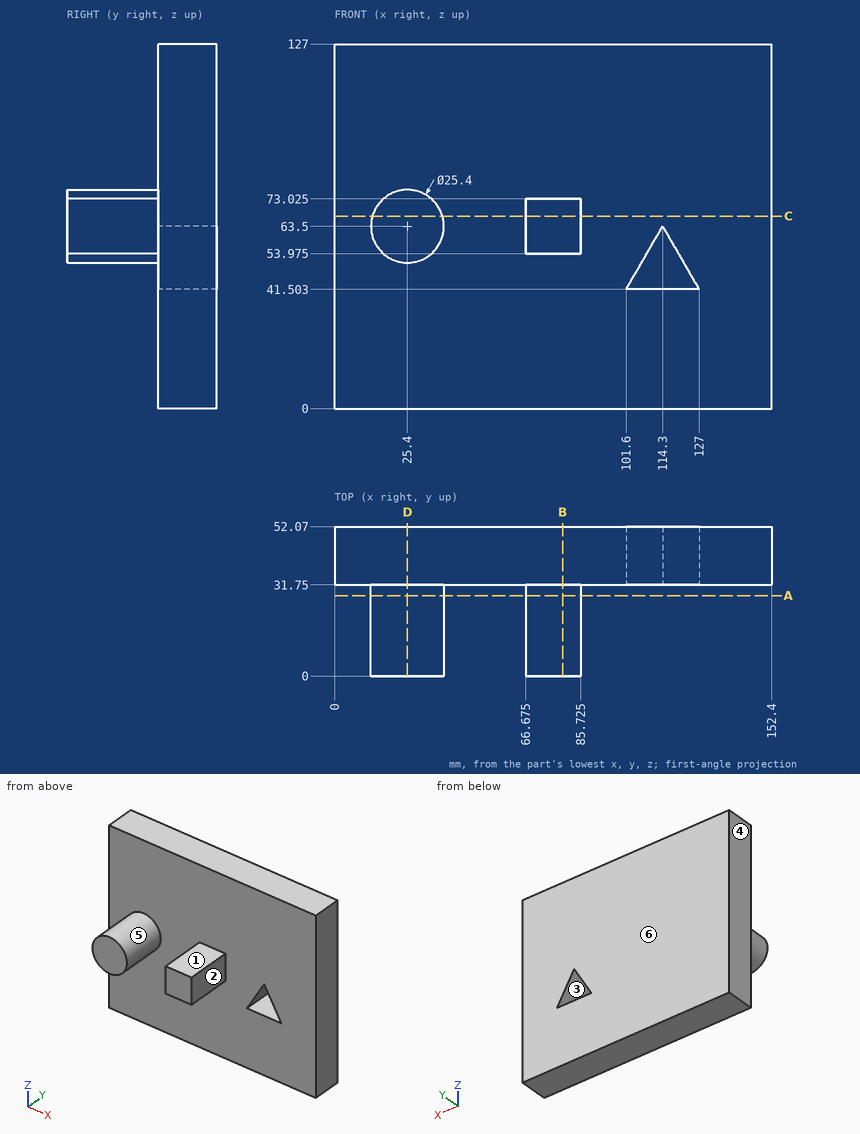
Part print with two shaded views. Sizes in mm from the minimum x, y, z corner. A direction names the side the tool comes from. Coordinates: 2 decimals unless noted, no trailing zeros. Order: outer loops, then holes, each group sorted by start corner. A loop starts at its lowest first (then second) coordinate and runs counter-clockwise, first axis right, second up. Notation, with made-up numbers: (87.25, 85.5) - (135.25, 85.5) arc R14 ccw to (135.25, 112.5) - close; hole circle Ø2 at (1, 18.5). An arc over 180 degrees is marked (long way). Answer in a Markdown table with one row per item.
1. 3-axis set-ups, long thin cutter, end or side, ignore diameter. For the marked faces 1, 2 and 3: which of +Z, -Z, +X, -X, +Y, -Y reach the whole face in a straight line?
Answer:
| item | result |
|---|---|
| face 1 | +Z, +X, -Y |
| face 2 | +Z, -Z, +X, -Y |
| face 3 | +Y, -Y |
2. Pull direction X, two halves, no side cores. Call the marked faces 4, 5 and 6: +X half, -X half, draft (parallel to the pull), parting line (faces both ways), or undercut.
Answer:
| item | result |
|---|---|
| face 4 | -X half |
| face 5 | undercut |
| face 6 | draft |
3. Slice it at D-D, the plane x = 25.4. List the corners of the cut face in (y, z), then the cut area to 3 significant figures.
Answer:
| item | result |
|---|---|
| outline | (0, 50.8) - (31.75, 50.8) - (31.75, 0) - (52.07, 0) - (52.07, 127) - (31.75, 127) - (31.75, 76.2) - (0, 76.2) - close |
| area | 3,390 mm² |
4. Slice it at A-A, the plane y = 28. List the corners of the cut face in (x, z) (3 decimals).
Answer:
| item | result |
|---|---|
| outline | circle Ø25.4 at (25.4, 63.5); (66.675, 53.975) - (85.725, 53.975) - (85.725, 73.025) - (66.675, 73.025) - close |
5. Slice it at C-C, the plane z = 67. List the corners of the cut face in (x, y) (3 decimals).
Answer:
| item | result |
|---|---|
| outline | (0, 31.75) - (13.192, 31.75) - (13.192, 0) - (37.608, 0) - (37.608, 31.75) - (66.675, 31.75) - (66.675, 0) - (85.725, 0) - (85.725, 31.75) - (152.4, 31.75) - (152.4, 52.07) - (0, 52.07) - close |
6. Flat gauge pins, fed straight in: P1, Ø5, axis at x = 91.5, z = 65.5, coming from the -Y side; P2, Ø15, axis at y = 11.5, z = 60.5, coming from the -X side; P3, Ø9.5, axis at x = 74, y = 12.5, coming from the -Z side (3 decimals). Where does each tip first touch, or does it go through?
Answer:
| item | result |
|---|---|
| P1 | y = 31.75 |
| P2 | x = 12.7 |
| P3 | z = 53.975 |
7. Drill centre lines: L1, parallel to X at y = 13, z = 67.5 (1 decimal); L2, parallel to Z at x = 81, y = 15 (3 decimals); L3, parallel to X at y = 15.5, z = 64 (3 decimals). Where is each one in solid material? Low to high. Write a range as from..to.
Answer:
| item | result |
|---|---|
| L1 | 13.3..37.5, 66.7..85.7 |
| L2 | 53.975..73.025 |
| L3 | 12.71..38.09, 66.675..85.725 |
8. Slice it at B-B, the plane x = 79.5. List the corners of the cut face in (y, z) (3 decimals), then the cut area to 3 significant figures.
Answer:
| item | result |
|---|---|
| outline | (0, 53.975) - (31.75, 53.975) - (31.75, 0) - (52.07, 0) - (52.07, 127) - (31.75, 127) - (31.75, 73.025) - (0, 73.025) - close |
| area | 3,190 mm² |
